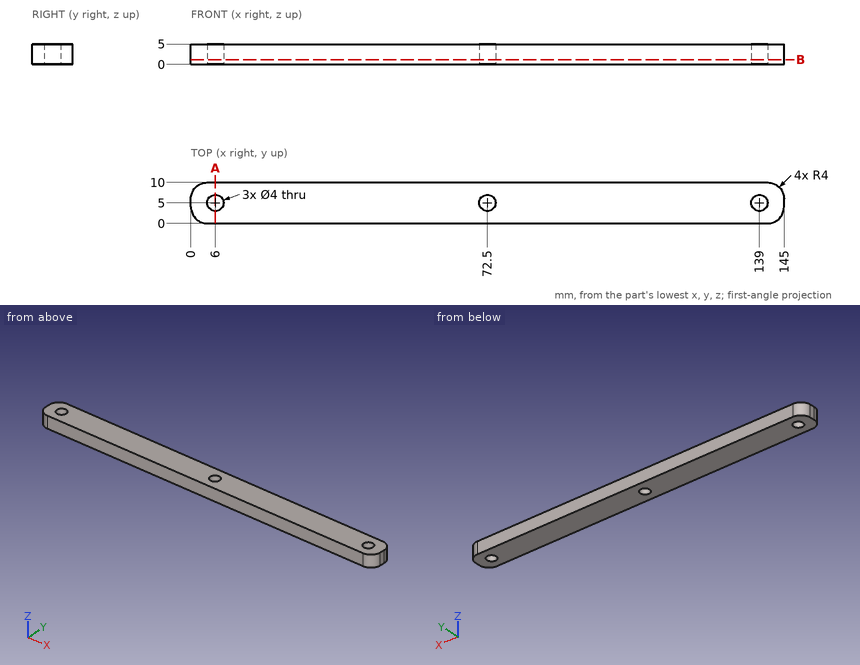
Part print with two shaded views. Sizes in mm from the minimum x, y, z corner. Round coordinates to 2 decimals unless told otherwise and drop trailing zeros. Order: outer loops, then holes, each group sorted by start corner. A loop starts at its lowest first (then second) coordinate and runs counter-clockwise, first axis right, second up. Notation, with made-up numbers: (3, 76.25) -> (15, 76.25) arc R17 cw to (15, 96.25) -> close; hole circle Ø9 at (-32, -12.5). An arc over 180 degrees is marked (long way). One line per question, with ' | ' between items.
Q1. Slice it at A-A (x = 6). Write the cut outline in (y, z), then the cut area to 3 significant figures.
Completed:
outline: (0, 0) -> (3, 0) -> (3, 5) -> (0, 5) -> close; (7, 0) -> (10, 0) -> (10, 5) -> (7, 5) -> close | area: 30.0 mm^2
Q2. Probe probe 1 along X at (y, z) = (5.25, 3.35); probe 2 along Y at (x, z) = (6, 3.7); probe 3 along X at (y, z) = (4.5, 3.2). List the from-to ranges inside material, lowest first.
Completed:
probe 1: x = 0 to 4.02, 7.98 to 70.52, 74.48 to 137.02, 140.98 to 145 | probe 2: y = 0 to 3, 7 to 10 | probe 3: x = 0 to 4.06, 7.94 to 70.56, 74.44 to 137.06, 140.94 to 145
Q3. Slice it at B-B (z = 1.15). Write the cut outline in (x, y).
Completed:
outline: (0, 4) arc R4 ccw to (4, 0) -> (141, 0) arc R4 ccw to (145, 4) -> (145, 6) arc R4 ccw to (141, 10) -> (4, 10) arc R4 ccw to (0, 6) -> close; hole circle Ø4 at (6, 5); hole circle Ø4 at (72.5, 5); hole circle Ø4 at (139, 5)
